Autodesk Inventor part; units mm, degrees
ref_plane "YZ Plane" through (0, 0, 0) normal (1, 0, 0) x (0, 1, 0)
ref_plane "XZ Plane" through (0, 0, 0) normal (0, 1, 0) x (-1, 0, 0)
ref_plane "XY Plane" through (0, 0, 0) normal (0, 0, 1) x (1, 0, 0)
sketch "Sketch1" plane through (0, 0, 0) normal (0, 1, 0) x (-1, 0, 0)
  line L0 (17.0295, 14.999) -> (-8.3705, 14.999)
  line L1 (-8.3705, 14.999) -> (-8.3705, -10.401)
  line L2 (-8.3705, -10.401) -> (17.0295, -10.401)
  line L3 (17.0295, -10.401) -> (17.0295, 14.999)
  line L4 (15.442, -8.8135) -> (-6.783, -8.8135)
  line L5 (-6.783, -8.8135) -> (-6.783, 13.4115)
  line L6 (-6.783, 13.4115) -> (15.442, 13.4115)
  line L7 (15.442, 13.4115) -> (15.442, -8.8135)
  point P0 (0, 0)
  dimension "d0" = 25.4
  dimension "d1" = 25.4
  dimension "d4" = 1.5875
  dimension "d5" = 1.5875
  dimension "d6" = 1.5875
  dimension "d7" = 1.5875
extrude "Extrusion2" add sketch "Sketch1" along normal blind 990.6
sketch "Sketch6" plane through (8.3705, 0, 14.999) normal (1, 0, 0) x (0, 0, -1)
  line L0 (25.4, 0) -> (25.4, 990.6)
  line L1 (0, 0) -> (25.4, 0)
  point P0 (14.999, 0)
  point P1 (12.7, 38.1)
  dimension "d46" = 12.7
  dimension "d47" = 38.1
hole "Hole5" at (8.3705, 38.1, 2.299) direction (-1, 0, 0) diameter 9.5758 depth 25.4 tip angle 118
sketch "Sketch7" plane through (8.3705, 0, 14.999) normal (1, 0, 0) x (0, 0, -1)
  line L0 (25.4, 0) -> (25.4, 990.6)
  line L1 (0, 990.6) -> (25.4, 990.6)
  point P0 (14.999, 0)
  point P1 (12.7, 965.2)
  dimension "d55" = 12.7
  dimension "d56" = 25.4
hole "Hole6" at (8.3705, 965.2, 2.299) direction (-1, 0, 0) diameter 9.5758 depth 25.4 tip angle 118
sketch "Sketch8" plane through (8.3705, 0, 14.999) normal (1, 0, 0) x (0, 0, -1)
  line L0 (0, 0) -> (25.4, 0)
  line L1 (25.4, 0) -> (25.4, 990.6)
  point P0 (14.999, 0)
  point P1 (12.7, 101.6)
  point P2 (12.7, 127)
  point P3 (12.7, 152.4)
  dimension "d64" = 25.4
  dimension "d65" = 25.4
  dimension "d66" = 101.6
  dimension "d67" = 12.7
  dimension "d68" = 0
  dimension "d69" = 0
hole "Hole7" at (8.3705, 101.6, 2.299) at (8.3705, 127, 2.299) at (8.3705, 152.4, 2.299) direction (-1, 0, 0) diameter 4.826 depth 25.4 tip angle 118
sketch "Sketch9" plane through (-17.0295, 0, 14.999) normal (0, 0, 1) x (1, 0, 0)
  line L0 (25.4, 0) -> (25.4, 990.6)
  line L1 (0, 990.6) -> (25.4, 990.6)
  line L2 (0, 0) -> (0, 990.6)
  point P0 (17.0295, 0)
  point P1 (19.05, 984.25)
  point P2 (6.35, 971.55)
  point P3 (19.05, 958.85)
  point P4 (6.35, 946.15)
  dimension "d77" = 6.35
  dimension "d78" = 6.35
  dimension "d79" = 6.35
  dimension "d80" = 6.35
  dimension "d81" = 6.35
  dimension "d82" = 19.05
  dimension "d83" = 25.4
  dimension "d84" = 25.4
hole "Hole8" at (2.0205, 984.25, 14.999) at (-10.6795, 971.55, 14.999) at (2.0205, 958.85, 14.999) at (-10.6795, 946.15, 14.999) direction (0, 0, -1) diameter 4.7625 depth 25.4 tip angle 118
sketch "Sketch10" plane through (-17.0295, 0, 14.999) normal (0, 0, 1) x (1, 0, 0)
  line L0 (25.4, 0) -> (25.4, 990.6)
  line L1 (0, 0) -> (0, 990.6)
  line L2 (0, 0) -> (25.4, 0)
  point P0 (17.0295, 0)
  point P1 (6.35, 69.85)
  point P2 (19.05, 57.15)
  point P3 (6.35, 44.45)
  point P4 (19.05, 31.75)
  dimension "d92" = 6.35
  dimension "d93" = 6.35
  dimension "d94" = 6.35
  dimension "d95" = 6.35
  dimension "d96" = 25.4
  dimension "d97" = 25.4
  dimension "d98" = 31.75
  dimension "d99" = 44.45
hole "Hole9" at (-10.6795, 69.85, 14.999) at (2.0205, 57.15, 14.999) at (-10.6795, 44.45, 14.999) at (2.0205, 31.75, 14.999) direction (0, 0, -1) diameter 4.7625 depth 25.4 tip angle 118
equation "\"d0\" = ElvBeamWidth"
equation "\"d1\" = ElvBeamWidth"
equation "\"d4\" = ElvWallWidth"
equation "\"d5\" = ElvWallWidth"
equation "\"d6\" = ElvWallWidth"
equation "\"d7\" = ElvWallWidth"
equation "\"d8\" = ElvFrontBeamLength"
equation "\"ElvMiddleBeamLength\" = 990.6"
equation "\"ElvWallWidth\" = 1.5875"
equation "\"ElvFrontBeamLength\" = 990.6"
equation "\"ElvEndEffectLength\" = 431.8"
equation "\"ElvCrossBeamLength\" = 304.8"
equation "\"ElvBeamWidth\" = 25.4"
equation "\"ElvFrontBeamLength_1\" = 1066.8"
equation "\"ElvFixedBeamLength\" = 990.6"
equation "\"ElvDelFrontTabLength\" = 6.35"
equation "\"ElvDelDepth\" = 6.35"
equation "\"ElvDelHeight\" = 101.6"
equation "\"ElvDelWidth\" = 18.542"
equation "\"ElvTopBeamLength\" = 457.2"
equation "\"ElvHoleFromBottom\" = 38.1"
equation "\"ElvHoleFromMid\" = 38.1"
equation "\"ElvHoleFromFixed\" = 50.8"
equation "\"ElvHoleFromFront\" = 25.4"
equation "\"ElvRivetPlateLength\" = 76.2"
equation "\"ElvDelMiddleTabLength\" = 6.35"
properties part number "ElvFrontBeam" material "Aluminum 6061"
Source: CAD feature listing. Evaluate the final solid. Frame: model axes, mm. A direction names the side the tool comes from. Coordinates: 2 decimals unless noted, no trailing zeros. Loops run counter-clockwise (first coordinate to the right, second up) from the corner with the lowest first, then second, coordinate; pieces in that order, holes last. Notation, with made-up numbers: (8.5, 23.25) - (39.5, 23.25) arc R21 ccw to (39.5, 49.25) - close; hole circle Ø3 at (49, 44.25). An arc over 180 degrees is marked (long way). Return JSON: item names as keys, results as strings.
Q1. Section A-A, the plane y = 929. Return loops of the section in (x, z).
Results:
{"outline": "(-17.03, -10.4) - (8.37, -10.4) - (8.37, 15) - (-17.03, 15) - close; hole (-15.44, -8.81) - (6.78, -8.81) - (6.78, 13.41) - (-15.44, 13.41) - close"}
Q2. Contact query for a flat-ended pin moving along its axis: P1, Ø4.5, axis at x = -10.68, y = 971.55, coming from the -Z side. Output: stop coordinate, or through.
Results:
{"P1": "through"}
Q3. Material intervals for line 1 along X through (y, z) = (57.15, -9.55); line 2 along X through (y, z) = (334, 9); line 3 along Z through (x, y) = (-6.5, 310.5), sorted ascending.
Results:
{"line 1": "-17.03 to -0.36, 4.4 to 8.37", "line 2": "-17.03 to -15.44, 6.78 to 8.37", "line 3": "-10.4 to -8.81, 13.41 to 15"}
Q4. Mould query, pull axis X, two halves, no side actions, for faces 1 (the flat face through (-15.442, 488, 2)), 2 (the flat face through (-17.03, 488, 2)), 3 (the flat face through (7, 990.6, 2)). Classes: released by +X, released by -X, zero draft, split by the parting line, or undercut.
Results:
{"face 1": "undercut", "face 2": "released by -X", "face 3": "zero draft"}
Q5. Access query for faces 4 (the flat face through (-4, 488, -10.401)), 5 (the flat face through (6.783, 488, 2)). Directions: +Z, -Z, +X, -X, +Y, -Y. A direction counts if a zero-diameter tool reaches every point of the face in a straight line with its end or side. Return the directions, or none.
Results:
{"face 4": "-Z, +X, -X, +Y, -Y", "face 5": "+Y, -Y"}
